from build123d import *

# Parameters (mm, degrees)
F0_W    = 32.086309
F0_H    = 76.2
F3_D    = 50.8
F4_SIZE = 2.54


with BuildPart() as f1:
    # F0 (on Front) → F1 (revolve)
    with BuildSketch(Plane.XZ):
        Polygon((0, 44.45), (0, 38.1), (32.086309, 38.1), (38.1, 38.1), (38.1, 44.45), align=None)
        with Locations((16.043154, 0)):
            Rectangle(F0_W, F0_H)
        Polygon((32.086309, -38.1), (0, -38.1), (0, -44.45), (38.1, -44.45), (38.1, -38.1), align=None)
    revolve(axis=Axis((0, 0, 0), (0, 0, -1)))

    # F3 (through all)
    with Locations(Plane.XY.offset(44.45)):
        with Locations((0, 0)):
            Hole(F3_D / 2)

    # F4
    f4_edges = [f1.edges().sort_by_distance(p)[0] for p in [
        (-38.1, 0, 44.45),
        (-38.1, 0, -44.45),
    ]]
    chamfer(f4_edges, length=F4_SIZE)


solid = f1.part
Geometry: final body of the model. Coordinates: model frame, mm. A direction names the side the tool comes from. Round coordinates to 2 decimals unless told otherwise and drop trailing zeros. Loops run counter-clockwise (first coordinate to the right, second up) from the corner with the lowest first, then second, coordinate; pieces in that order, holes last. Notation, with made-up numbers: (62, 69.25) -> (92, 69.25) arc R28 cw to (92, 97.25) -> close; hole circle Ø3 at (47.5, 62). An arc over 180 degrees is marked (long way). One line per question, with ' | ' between items. Start each with the question number.
1. Contact query for flat-ended pins moving along their axis: pin 1 (5 mm diameter, centred on x = -8.5, z = -17.5, fed in from +Y); pin 2 (1 mm diameter, centred on x = -7, z = -3.5, fed in from +Y); pin 3 (8 mm diameter, centred on y = -26, z = -20.5, fed in from -X). Output: stop coordinate, or through.
2. Line query: line 1 along Y through (x, z) = (0, 15.5); line 2 along Y through (x, z) = (0.5, -38.5); line 3 along Z through (x, y) = (-6.5, 33.5). Output: solid intervals per line, ascending. Write a range as [from, to].
3. Mould query, pull axis Z, two halves, no side actions, for faces 3 (the face through (30.605, -9.638, 0.533)), 4 (the face through (-17, 28, -38.1)), 5 (the face through (-30.235, 23.183, -39.978)), 6 (the face through (-24.2, -8.4, 44.45)). Classes: pulls with the +Z half, pulls with the -Z half, needs draft (parallel to the pull), parting line crosses it, or undercut.
4. Section A-A on x = 0. Output: boundary loops of the cut face in (y, z), and give its area (3 significant figures).
5. Section C-C on z = -7. Output: boundary loops of the cut face in (x, y), and give its area (3 significant figures).
6. Set-up query: faces 1 (the face through (17, 28, 38.1)), 2 (the face through (-7.74, 34.87, 44.29)). Return all of +Z, -Z, +X, -X, +Y, -Y with unobstructed straight access to the full face (end or side cutting, diameter ignored); none if empty.
Returned:
1) pin 1: stops at y = 31.52 | pin 2: stops at y = 31.42 | pin 3: stops at x = -23.36
2) line 1: y = [-32.09, -25.4], [25.4, 32.09] | line 2: y = [-38.1, -25.4], [25.4, 38.1] | line 3: z = [-44.45, -38.1], [38.1, 44.45]
3) face 3: undercut | face 4: undercut | face 5: needs draft | face 6: pulls with the +Z half
4) outline: (-38.1, -41.91) -> (-35.56, -44.45) -> (-25.4, -44.45) -> (-25.4, 44.45) -> (-35.56, 44.45) -> (-38.1, 41.91) -> (-38.1, 38.1) -> (-32.09, 38.1) -> (-32.09, -38.1) -> (-38.1, -38.1) -> close; (25.4, -44.45) -> (35.56, -44.45) -> (38.1, -41.91) -> (38.1, -38.1) -> (32.09, -38.1) -> (32.09, 38.1) -> (38.1, 38.1) -> (38.1, 41.91) -> (35.56, 44.45) -> (25.4, 44.45) -> close | area: 1,330 mm2
5) outline: circle Ø64.17 at (0, 0); hole circle Ø50.8 at (0, 0) | area: 1,210 mm2
6) face 1: none | face 2: +Z
